The model under review builds one solid part; all positions refer to its coordinate system, in mm. Face numbers are marked on the shaded views. A direction names the side the tool comes from. Round coordinates to 2 decimals unless told otherwise and drop trailing zeros. Order: outer loops, then holes, each group sorted by start corner. A loop starts at its lowest first (then second) coordinate and runs counter-clockwise, first axis right, second up.
1) To check wall thickness, follow L1, parallel to X at y = 39, z = -4.25 (3 decimals); L2, parallel to Y at x = 596.9, z = 1.6; L3, parallel to X at y = 304.8, z = 1.3. State the ranges of each line that lie inside material, in increasing order.
2) Clearance check with flat-ended pins moving along their axes: P1, Ø3, axis at x = 526, z = -4, coming from the +Y side; P2, Ø3, axis at x = 388, z = -16.5, coming from the +Y side; P3, Ø16.5, axis at x = 538.23, y = 280.5, coming from the -Z side. State where each tip first meets the part, or that it passes through.
3) Consider section A-A (y = -11). Give the boundary of the cut face in (x, z) (3 decimals).
4) Consider section B-B (x = 596.9). Give the boundary of the cut face in (y, z) (3 decimals).
5) Machinability: for the marked faces 1 and 2, which of the approach directions +Z, -Z, +X, -X, +Y, -Y give a long, thin tool a straight path to every point of the face, cutting with its end or side? Answer none if there is none.
6) Consider section C-C (z = -5.25). Give the boundary of the cut face in (x, y) (3 decimals).
Autodesk Inventor part; units mm, degrees
ref_plane "Work Plane1" through (0, 0, 0) normal (0, 0, 1) x (1, 0, 0)
ref_plane "YZ Plane" through (0, 0, 0) normal (1, 0, 0) x (0, 1, 0)
ref_plane "XZ Plane" through (0, 0, 0) normal (0, 1, 0) x (-1, 0, 0)
ref_plane "Work Plane1" through (0, 0, 0) normal (0, 0, 1) x (1, 0, 0)
sketch "Sketch1" plane through (0, 0, 0) normal (0, 0, 1) x (1, 0, 0)
  line L0 (0, 0) -> (63.5, 0)
  line L1 (63.5, 0) -> (63.5, 482.6)
  line L2 (63.5, 482.6) -> (0, 482.6)
  line L3 (0, 482.6) -> (0, 0)
  line L4 (63.5, 482.6) -> (63.5, 406.4)
  line L5 (63.5, 482.6) -> (139.7, 482.6) construction
  line L6 (63.5, 406.4) -> (-63.5, 406.4)
  line L7 (63.5, 406.4) -> (63.5, 304.8)
  line L8 (63.5, 406.4) -> (165.1, 406.4) construction
  line L9 (63.5, 304.8) -> (1409.7, 304.8)
  line L10 (63.5, 304.8) -> (596.9, 304.8)
  circle A0 centre (596.9, 304.8) radius 88.9
  circle A1 centre (596.9, 304.8) radius 6.35
  line L11 (596.9, 304.8) -> (1174.248, 304.8) construction
  line L12 (596.9, 304.8) -> (538.2336, 280.4996)
  circle A2 centre (538.2336, 280.4996) radius 6.35
  line L13 (596.9, 304.8) -> (614.4999, 312.0901)
  line L14 (596.9, 304.8) -> (615.95, 304.8) construction
  line L15 (614.4999, 312.0901) -> (619.36, 300.3568)
  line L16 (619.36, 300.3568) -> (63.5, 70.1121)
  line L17 (614.4999, 312.0901) -> (609.6398, 323.8234)
  line L18 (614.4999, 312.0901) -> (627.1999, 312.0901) construction
  line L19 (609.6398, 323.8234) -> (63.5, 97.6049)
  line L20 (63.5, 70.1121) -> (63.5, -183.8879)
  line L21 (63.5, 70.1121) -> (317.5, 70.1121) construction
  line L22 (63.5, -183.8879) -> (88.9, -183.8879)
  line L23 (88.9, -183.8879) -> (88.9, 80.6331)
  dimension "d0" = 63.5
  dimension "d1" = 482.6
  dimension "d2" = 76.2
  dimension "d3" = 90
  dimension "d4" = 127
  dimension "d5" = 90
  dimension "d6" = 101.6
  dimension "d7" = 90
  dimension "d8" = 1346.2
  dimension "d9" = 90
  dimension "d10" = 533.4
  dimension "d11" = 177.8
  dimension "d12" = 12.7
  dimension "d14" = 63.5
  dimension "d15" = 12.7
  dimension "d16" = 19.05
  dimension "d17" = 22.5
  dimension "d18" = 12.7
  dimension "d19" = 90
  dimension "d20" = 90
  dimension "d21" = 12.7
  dimension "d22" = 112.5
  dimension "d23" = 591.1375
  dimension "d24" = 90
  dimension "d25" = 254
  dimension "d26" = 90
  dimension "d27" = 25.4
  dimension "d28" = 90
  dimension "d29" = 90
extrude "Extrusion1" add sketch "Sketch1" along normal blind 25.4 contours L1 L16 L23 L22 L20 | L1 L19 A0 L16 | L19 L9 A1 L15 L16 A0 | L19 L17 L13 A1 L9 | L9 A1 L13 L15
sketch "Sketch2" plane through (0, 0, 25.4) normal (0, 0, 1) x (1, 0, 0)
  circle A0 centre (596.9, 304.8) radius 6.35
  line L0 (88.9, 80.6331) -> (619.36, 300.3568)
  line L1 (619.36, 300.3568) -> (609.6398, 323.8234)
  line L2 (609.6398, 323.8234) -> (63.5, 97.6049)
  line L3 (63.5, 97.6049) -> (63.5, -183.8879)
  line L4 (63.5, -183.8879) -> (88.9, -183.8879)
  line L5 (88.9, -183.8879) -> (88.9, 80.6331)
  line L6 (596.9, 304.8) -> (614.4999, 312.0901)
  line L7 (596.9, 304.8) -> (615.95, 304.8) construction
  line L8 (614.4999, 312.0901) -> (604.7797, 335.5567)
  line L9 (614.4999, 312.0901) -> (639.8999, 312.0901) construction
  line L10 (604.7797, 335.5567) -> (624.2201, 288.6236)
  line L11 (624.2201, 288.6236) -> (1203.6463, 288.6236) construction
  line L12 (604.7797, 335.5567) -> (1190.6567, 335.5567) construction
  line L13 (76.2, -183.8879) -> (101.6, -183.8879)
  line L14 (101.6, -183.8879) -> (50.8, -183.8879)
  line L15 (101.6, -183.8879) -> (101.6, 72.1473)
  line L16 (101.6, 72.1473) -> (624.2201, 288.6236)
  line L17 (604.7797, 335.5567) -> (50.8, 106.0907)
  line L18 (604.7797, 335.5567) -> (1204.4031, 335.5567) construction
  line L19 (50.8, 106.0907) -> (50.8, -183.8879)
  point P0 (0, 0)
  dimension "d32" = 22.5
  dimension "d33" = 25.4
  dimension "d34" = 112.5
  dimension "d35" = 50.8
  dimension "d36" = 0
  dimension "d39" = 25.4
  dimension "d40" = 50.8
  dimension "d42" = 157.5
extrude "Extrusion2" add sketch "Sketch2" against normal blind 25.4 contours L10 L16 L15 L13 L5 L0 | L2 L3 L14 L19 L17 L8
sketch "Sketch4" plane through (0, 0, 25.4) normal (0, 0, 1) x (1, 0, 0)
  line L0 (604.7797, 335.5567) -> (50.8, 106.0907)
  line L1 (50.8, 106.0907) -> (50.8, -183.8879)
  line L2 (50.8, -183.8879) -> (101.6, -183.8879)
  line L3 (101.6, -183.8879) -> (101.6, 72.1473)
  line L4 (76.2, -183.8879) -> (76.2, 116.6118)
  point P0 (0, 0)
extrude "Extrusion3" cut sketch "Sketch4" against normal blind 25.4
sketch "Sketch5" plane through (0, 0, 25.4) normal (0, 0, 1) x (1, 0, 0)
  line L0 (76.2, 116.6118) -> (76.2, -183.8879)
  line L1 (76.2, -183.8879) -> (101.6, -183.8879)
  line L2 (101.6, -183.8879) -> (101.6, 72.1473)
  line L3 (101.6, 72.1473) -> (624.2201, 288.6236)
  line L4 (624.2201, 288.6236) -> (604.7797, 335.5567)
  line L5 (604.7797, 335.5567) -> (76.2, 116.6118)
  circle A0 centre (538.2336, 280.4996) radius 6.35
  circle A1 centre (596.9, 304.8) radius 6.35
  line L6 (101.6, -183.8879) -> (98.425, -183.8879)
  line L7 (101.6, -183.8879) -> (104.775, -183.8879) construction
  line L8 (624.2201, 288.6236) -> (623.005, 291.5569)
  line L9 (624.2201, 288.6236) -> (627.3951, 288.6236) construction
  line L10 (623.005, 291.5569) -> (98.425, 74.2687)
  line L11 (98.425, 74.2687) -> (98.425, -183.8879)
  point P0 (0, 0)
  dimension "d61" = 3.175
  dimension "d62" = 180
  dimension "d63" = 3.175
  dimension "d64" = 112.5
  dimension "d65" = 90
extrude "Extrusion4" cut sketch "Sketch5" against normal blind 22.225 contours L5 L4 L10 L11 L1 L0
sketch "Sketch6" plane through (0, 0, 25.4) normal (0, 0, 1) x (1, 0, 0)
  line L0 (623.005, 291.5569) -> (98.425, 74.2687)
  line L1 (98.425, 74.2687) -> (98.425, -183.8879)
  line L2 (98.425, -183.8879) -> (101.6, -183.8879)
  line L3 (101.6, -183.8879) -> (101.6, 72.1473)
  line L4 (101.6, 72.1473) -> (624.2201, 288.6236)
  line L5 (624.2201, 288.6236) -> (623.005, 291.5569)
  point P0 (0, 0)
extrude "Extrusion5" add sketch "Sketch6" against normal blind 47.625
sketch "Sketch7" plane through (0, 0, 25.4) normal (0, 0, 1) x (1, 0, 0)
  line L0 (623.005, 291.5569) -> (98.425, 74.2687)
  line L1 (98.425, 74.2687) -> (98.425, -183.8879)
  line L2 (98.425, -183.8879) -> (101.6, -183.8879)
  line L3 (101.6, -183.8879) -> (101.6, 72.1473)
  line L4 (101.6, 72.1473) -> (624.2201, 288.6236)
  line L5 (624.2201, 288.6236) -> (623.005, 291.5569)
  point P0 (0, 0)
extrude "Extrusion6" cut sketch "Sketch7" against normal blind 22.225
properties part number "CatapultArmL-Left"
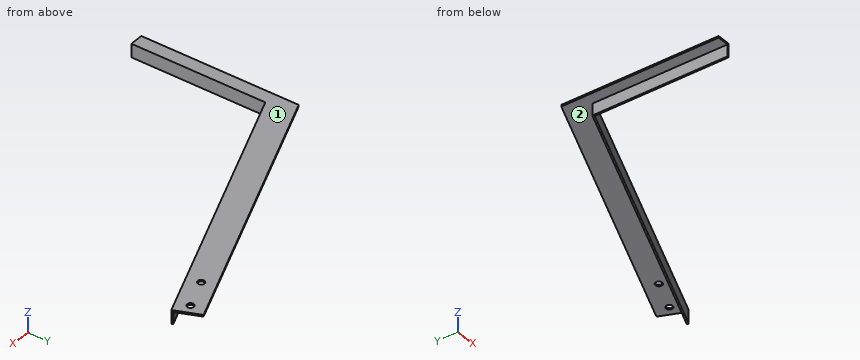
Answer below:
1. L1: x = 98.425 to 101.6
1. L2: y = 277.31 to 298.45, 311.15 to 332.29
1. L3: x = 530.53 to 590.55, 603.25 to 617.52
2. P1: stops at y = 252
2. P2: stops at y = 194.84
2. P3: stops at z = 0
3. outline: (76.2, 0) - (98.425, 0) - (98.425, -22.225) - (101.6, -22.225) - (101.6, 3.175) - (76.2, 3.175) - close
4. outline: (277.307, -22.225) - (280.744, -22.225) - (280.744, 0) - (298.45, 0) - (298.45, 3.175) - (277.307, 3.175) - close; (311.15, 0) - (332.293, 0) - (332.293, 3.175) - (311.15, 3.175) - close
5. face 1: +Z, +X, -X, +Y, -Y
5. face 2: -Z, -X, +Y
6. outline: (98.425, -183.888) - (101.6, -183.888) - (101.6, 72.147) - (624.22, 288.624) - (623.005, 291.557) - (98.425, 74.269) - close
